Build history of the part. All positions in model axes, mm. Round coordinates to 2 decimals unless told otherwise and drop trailing zeros. Write each loop counter-clockwise with the first axis right and the second up, starting at its lowest first coordinate (ties: lowest second). Pieces come first, ordered by that corner, then holes. Notation, with made-up numbers: (44, 50) -> (68, 50) arc R13 cw to (68, 69) -> close; hole circle Ø9 at (88.25, -34). An arc over 180 degrees is marked (long way). Answer as CSV lines item,"result".
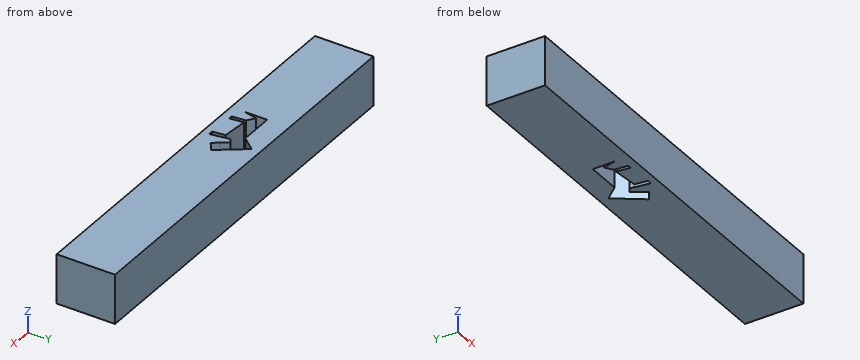
from build123d import *

# Parameters (mm, degrees)
F0_W     = 88.7035392225
F0_H     = 75.0795733184
F1_DEPTH = 609.6
F3_DEPTH = 75.0805733184


with BuildPart() as f1:
    # F0 (on Right) → F1 (new body)
    with BuildSketch(Plane.YZ):
        with Locations((10.8415391296, -13.1027223542)):
            Rectangle(F0_W, F0_H)
    extrude(amount=F1_DEPTH)

    # F2 (on face) → F3 (cut, through all)
    with BuildSketch(Plane.XY.offset(24.4370643049)):
        Polygon((250.0542104244, 21.7413976789), (198.4199732542, 21.7413976789), (198.4199732542, -12.5776519999), (203.0778974295, 7.6524470933), (214.2598032951, 0), (216.5598422289, -20.7415837795), (221.9552248716, -20.7415837795), (219.3950414658, 0), (257.3667168617, -3.4582386725), (259.7696781158, -22.5320160389), (266.5723860264, -22.5320160389), (261.9751274163, 6.5919420698), (268.5813307762, 11.1460844055), (276.2651473502, 0), (283.1545623022, -9.7264384601), (296.8862950802, 0), (266.9985592365, 42.1953424811), align=None)
    extrude(amount=-F3_DEPTH, mode=Mode.SUBTRACT)


solid = f1.part
1. Probe line 1 along X through (y, z) = (5.5, -30); line 2 along X through (y, z) = (-13.5, -42); line 3 along X through (y, z) = (0.5, -17). List the from-to ranges inside material, lowest first.
Results found:
line 1,"x = 0 to 198.42, 202.58 to 206.22, 262.15 to 272.47, 292.99 to 609.6"
line 2,"x = 0 to 215.76, 221.06 to 258.63, 265.15 to 609.6"
line 3,"x = 0 to 198.42, 201.43 to 213.53, 262.94 to 275.92, 296.53 to 609.6"
2. Cut at A-A, the plane z = 15. Write the cut outline in (x, y).
Results found:
outline,"(0, -33.51) -> (609.6, -33.51) -> (609.6, 55.19) -> (0, 55.19) -> close; hole (198.42, -12.58) -> (203.08, 7.65) -> (214.26, 0) -> (216.56, -20.74) -> (221.96, -20.74) -> (219.4, 0) -> (257.37, -3.46) -> (259.77, -22.53) -> (266.57, -22.53) -> (261.98, 6.59) -> (268.58, 11.15) -> (276.27, 0) -> (283.15, -9.73) -> (296.89, 0) -> (267, 42.2) -> (250.05, 21.74) -> (198.42, 21.74) -> close"
3. Drop a flat-ended pin along its axis: pin 1 Ø5 at (y, z) = (-9, -31.5) entering from -X. Give the stop position or say it passes through.
Results found:
pin 1,"stops at x = 0"
